Part model, mm, in its own coordinate system. Round coordinates to 2 decimals unless told otherwise and drop trailing zeros. Write each loop counter-clockwise with the first axis right and the second up, starting at its lowest first coordinate (ties: lowest second). Pieces come first, ordered by that corner, then holes.
1) Drill centre lines: L1, parallel to Y at x = 18.5, z = 3.7; L2, parallel to X at y = 25, z = 4.4; L3, parallel to X at y = -27, z = 2.5. Where is each one in solid material? Low to high.
2) Saw through at A-A on z = 1.15. Write the cut outline in (x, y), and give its area (3 significant figures).
3) Saw through at B-B on x = 31.5. Write the cut outline in (y, z), and give its area (3 significant figures).
4) Saw through at C-C on y = 30. Write the cut outline in (x, z).
5) Pull direction X, two halves, no side cores. Call faces 1 (the cylindrical face through (55.49, -21.95, 2.46)), 2 (the cylindrical face through (16.07, 38.13, 2.46)), 3 (the flat face through (31, -16, 0)): +X half, -X half, draft (parallel to the pull), parting line (faces both ways), or undercut.
6) Flat gauge pins, fed straight in: pin 1 (1.5 mm diameter, centred on y = -28.5, z = 2, fed in from -X); pin 2 (3 mm diameter, centred on x = 35, z = 0.5, fed in from +Y). Where does each tip first touch, or does it go through?
```python
from build123d import *

# Parameters (mm, degrees)
SKETCH1_R           = 1.7
BOSS_EXTRUDE1_DEPTH = 5


with BuildPart() as part:
    # Sketch1 → Boss-Extrude1 (new body)
    with BuildSketch(Plane.XY):
        with BuildLine():
            Line((9.571131615, 22.290661788), (12.45890696, -7.549683437))
            ThreePointArc((12.45890696, -7.549683437), (12.772506188, -8.872231039), (13.430707906, -10.06145227))
            Line((13.430707906, -10.06145227), (46.762768529, -54.65745062))
            ThreePointArc((46.762768529, -54.65745062), (49.46823245, -56.492242481), (52.729148127, -56.263277104))
            Line((52.729148127, -56.263277104), (61.868035374, -52.365810483))
            ThreePointArc((61.868035374, -52.365810483), (64.497484035, -49.747459847), (64.598320481, -46.038067399))
            Line((64.598320481, -46.038067399), (56.204499393, -23.254838732))
            ThreePointArc((56.204499393, -23.254838732), (55.474314099, -21.932746284), (54.382663092, -20.889004416))
            Line((54.382663092, -20.889004416), (28.713394846, -2.896526673))
            Line((28.713394846, -2.896526673), (20.09267624, 42.882461783))
            ThreePointArc((20.09267624, 42.882461783), (18.924854223, 45.269094952), (16.699240102, 46.720462558))
            Line((16.699240102, 46.720462558), (16.091332484, 46.914475628))
            ThreePointArc((16.091332484, 46.914475628), (11.621640502, 46.18856761), (9.571131615, 42.151179571))
            Line((9.571131615, 42.151179571), (9.571131615, 22.290661788))
        make_face()
        with Locations((15.155921835, 36.698515682)):
            Circle(SKETCH1_R, mode=Mode.SUBTRACT)
        with Locations((19.648657186, -7.364112555)):
            Circle(SKETCH1_R, mode=Mode.SUBTRACT)
    extrude(amount=BOSS_EXTRUDE1_DEPTH)


solid = part.part
```
Completed:
1. L1: y = -16.84 to -8.62, -6.11 to 45.69
1. L2: x = 9.57 to 23.46
1. L3: x = 26.09 to 57.58
2. outline: (9.57, 22.29) - (12.46, -7.55) arc R5 ccw to (13.43, -10.06) - (46.76, -54.66) arc R5 ccw to (52.73, -56.26) - (61.87, -52.37) arc R5 ccw to (64.6, -46.04) - (56.2, -23.25) arc R5 ccw to (54.38, -20.89) - (28.71, -2.9) - (20.09, 42.88) arc R5 ccw to (16.7, 46.72) - (16.09, 46.91) arc R5 ccw to (9.57, 42.15) - close; hole circle Ø3.4 at (15.16, 36.7); hole circle Ø3.4 at (19.65, -7.36)
2. area: 2,040 mm2
3. outline: (-34.24, 0) - (-4.85, 0) - (-4.85, 5) - (-34.24, 5) - close
3. area: 147 mm2
4. outline: (9.57, 0) - (22.52, 0) - (22.52, 5) - (9.57, 5) - close
5. face 1: +X half
5. face 2: undercut
5. face 3: draft
6. pin 1: stops at x = 26.65
6. pin 2: stops at y = -6.25
